```python
from build123d import *

# Parameters (mm, degrees)
BOSS_EXTRUDE1_DEPTH = 3
CUT_EXTRUDE1_DEPTH  = 72.651936471
SKETCH3_W           = 3
SKETCH3_H           = 15
CUT_EXTRUDE2_DEPTH  = 72.651936471
SKETCH4_R           = 1.6
CUT_EXTRUDE3_DEPTH  = 72.651936471


with BuildPart() as part:
    # Sketch1 → Boss-Extrude1 (new body)
    with BuildSketch(Plane(origin=(0, 0, 0), x_dir=(1, 0, 0), z_dir=(0, 1, 0))):
        Polygon((-65, 27), (-52.5, 27), (-52.5, 30), (-37.5, 30), (-37.5, 27), (-22.5, 27), (-22.5, 30), (-7.5, 30), (-7.5, 27), (7.5, 27), (7.5, 30), (22.5, 30), (22.5, 27), (37.5, 27), (37.5, 30), (52.5, 30), (52.5, 27), (65, 27), (65, -27), (52.5, -27), (52.5, -30), (37.5, -30), (37.5, -27), (22.5, -27), (22.5, -30), (7.5, -30), (7.5, -27), (-7.5, -27), (-7.5, -30), (-22.5, -30), (-22.5, -27), (-37.5, -27), (-37.5, -30), (-52.5, -30), (-52.5, -27), (-65, -27), align=None)
    extrude(amount=BOSS_EXTRUDE1_DEPTH)

    # Sketch2 → Cut-Extrude1 (cut, through all)
    with BuildSketch(Plane(origin=(0, 3, 0), x_dir=(1, 0, 0), z_dir=(0, 1, 0))):
        with BuildLine():
            Line((-55, 1.6), (-50, 1.6))
            ThreePointArc((-50, 1.6), (-48.4, 0), (-50, -1.6))
            Line((-50, -1.6), (-55, -1.6))
            ThreePointArc((-55, -1.6), (-56.6, 0), (-55, 1.6))
        make_face()
        with BuildLine():
            Line((55, 1.6), (50, 1.6))
            ThreePointArc((50, 1.6), (48.4, 0), (50, -1.6))
            Line((50, -1.6), (55, -1.6))
            ThreePointArc((55, -1.6), (56.6, 0), (55, 1.6))
        make_face()
        with BuildLine():
            Line((-55, 19.6), (-50, 19.6))
            ThreePointArc((-50, 19.6), (-48.4, 18), (-50, 16.4))
            Line((-50, 16.4), (-55, 16.4))
            ThreePointArc((-55, 16.4), (-56.6, 18), (-55, 19.6))
        make_face()
        with BuildLine():
            Line((-55, -16.4), (-50, -16.4))
            ThreePointArc((-50, -16.4), (-48.4, -18), (-50, -19.6))
            Line((-50, -19.6), (-55, -19.6))
            ThreePointArc((-55, -19.6), (-56.6, -18), (-55, -16.4))
        make_face()
        with BuildLine():
            Line((55, 19.6), (50, 19.6))
            ThreePointArc((50, 19.6), (48.4, 18), (50, 16.4))
            Line((50, 16.4), (55, 16.4))
            ThreePointArc((55, 16.4), (56.6, 18), (55, 19.6))
        make_face()
        with BuildLine():
            Line((55, -16.4), (50, -16.4))
            ThreePointArc((50, -16.4), (48.4, -18), (50, -19.6))
            Line((50, -19.6), (55, -19.6))
            ThreePointArc((55, -19.6), (56.6, -18), (55, -16.4))
        make_face()
    extrude(amount=-CUT_EXTRUDE1_DEPTH, mode=Mode.SUBTRACT)

    # Sketch3 → Cut-Extrude2 (cut, through all)
    with BuildSketch(Plane(origin=(0, 3, 0), x_dir=(1, 0, 0), z_dir=(0, 1, 0))):
        Rectangle(SKETCH3_W, SKETCH3_H)
    extrude(amount=-CUT_EXTRUDE2_DEPTH, mode=Mode.SUBTRACT)

    # Sketch4 → Cut-Extrude3 (cut, through all)
    with BuildSketch(Plane.XZ):
        with Locations(Location((-28.1, -0.65, 0), (0, 0, 270))):
            Circle(SKETCH4_R)
        with Locations(Location((-28.1, -18.35, 0), (0, 0, 270))):
            Circle(SKETCH4_R)
    cut_extrude3 = extrude(amount=-CUT_EXTRUDE3_DEPTH, mode=Mode.SUBTRACT)

    # Mirror1: Cut-Extrude3 across plane
    add(cut_extrude3.mirror(Plane(origin=(0, 0, 0), x_dir=(0, 0, 1), z_dir=(1, 0, 0))), mode=Mode.SUBTRACT)


solid = part.part
```
Could you check a few things on this model? Use its own coordinates, in mm. A direction names the side the tool comes from. Round coordinates to 2 decimals unless told otherwise and drop trailing zeros. Loops run counter-clockwise (first coordinate to the right, second up) from the corner with the lowest first, then second, coordinate; pieces in that order, holes last. Notation, with made-up numbers: (27, 44.25) - (53, 44.25) arc R21 cw to (53, 79.25) - close; hole circle Ø10 at (-22, 0.5). An arc over 180 degrees is marked (long way). Answer in a Markdown table with one row per item. Add a question column.
(1) If we section it at B-B (y = 1.55): State how many separate pieces and enclosed holes the cut face has, plus the area to 3 significant figures.
(2) If we section it at C-C (x = -36): Please give me the cut outline in (y, z).
(3) For faces 1 (the face through (-59, 1, 27)), 2 (the face through (30, 1, -27)), 3 (the face through (52, 2, 1.6)), 4 (the face through (22.5, 1, 28)), which set-ups out of +Z, -Z, +X, -X, +Y, -Y let a thin tool reach every point of the face, with its end or its side?
(4) I'm going to push flat-ended pins straight in: pin 1 (0.9 mm diameter, centred on x = -27, y = 1.5, fed in from +Z); pin 2 (1.5 mm diameter, centred on x = 55.5, y = 1, fed in from -Z); pin 3 (1.9 mm diameter, centred on x = 28.1, z = -0.65, fed in from -Y); pin 4 (0.9 mm diameter, centred on y = 1, z = -28.5, fed in from -X). Where does each tip first touch, or does it pass through?
(5) I need wall thicknesses on line 1 along Z through (x, y) = (28.1, 1.1); line 2 along X through (y, z) = (2.2, -2.5); line 3 along X through (y, z) = (2.55, 17). Which ranges of each line are inside material? Lowest first, please.
(6) If we section it at A-A (z = 18): Please give me the cut outline in (x, y).
(7) If we mould it in two halves opening along Z, with no side actions, what happens to faces 5 (the face through (-48.4, 1.5, 0)), 6 (the face through (52.5, 1, 28)), 7 (the face through (15, 1, -30))? For each: pulls with the +Z half, pulls with the -Z half, needs draft (parallel to the pull), parting line crosses it, or undercut.
Model answer:
| question | item | result |
|---|---|---|
| 1 | separate pieces | 1 |
| 1 | enclosed holes | 11 |
| 1 | area | 7,160 mm² |
| 2 | outline | (0, -27) - (3, -27) - (3, 27) - (0, 27) - close |
| 3 | face 1 | +Z, -X, +Y, -Y |
| 3 | face 2 | -Z, +Y, -Y |
| 3 | face 3 | +Y, -Y |
| 3 | face 4 | +Z, +Y, -Y |
| 4 | pin 1 | stops at z = 27 |
| 4 | pin 2 | stops at z = -27 |
| 4 | pin 3 | passes through |
| 4 | pin 4 | stops at x = -52.5 |
| 5 | line 1 | z = -27 to -19.95, -16.75 to -2.25, 0.95 to 27 |
| 5 | line 2 | x = -65 to -1.5, 1.5 to 65 |
| 5 | line 3 | x = -65 to -56.25, -48.75 to 48.75, 56.25 to 65 |
| 6 | outline | (-65, 0) - (-56.6, 0) - (-56.6, 3) - (-65, 3) - close; (-48.4, 0) - (48.4, 0) - (48.4, 3) - (-48.4, 3) - close; (56.6, 0) - (65, 0) - (65, 3) - (56.6, 3) - close |
| 7 | face 5 | undercut |
| 7 | face 6 | needs draft |
| 7 | face 7 | pulls with the -Z half |
